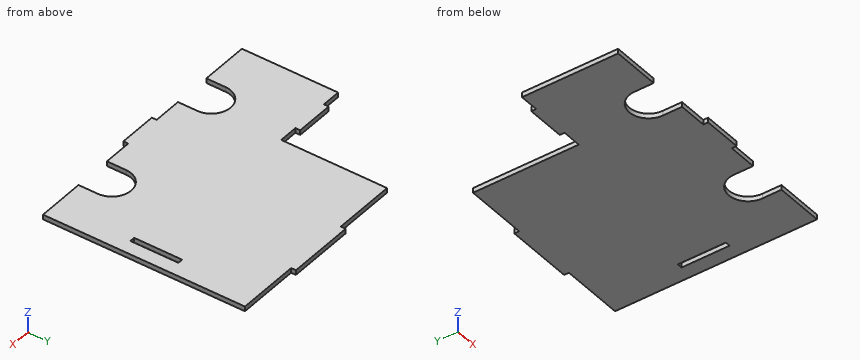
Autodesk Inventor part; units mm, degrees
ref_plane "YZ Plane" through (0, 0, 0) normal (1, 0, 0) x (0, 1, 0)
ref_plane "XZ Plane" through (0, 0, 0) normal (0, 1, 0) x (-1, 0, 0)
ref_plane "XY Plane" through (0, 0, 0) normal (0, 0, 1) x (1, 0, 0)
sketch "Sketch1" plane through (0, 0, 0) normal (0, 0, 1) x (1, 0, 0)
  line L0 (0, 0) -> (0, 100)
  line L1 (0, 100) -> (80, 100)
  line L2 (80, 100) -> (80, 210)
  line L3 (80, 210) -> (280, 210)
  line L4 (280, 210) -> (280, 0)
  line L5 (0, 0) -> (50, 0)
  line L6 (50, 0) -> (50, 20)
  arc A0 (90, 20) -> (50, 20) centre (70, 20) ccw
  line L7 (90, 20) -> (90, 0)
  line L8 (140, 0) -> (140, 210) construction
  line L9 (90, 0) -> (140, 0)
  line L10 (280, 0) -> (230, 0)
  line L11 (230, 0) -> (230, 20)
  arc A1 (230, 20) -> (190, 20) centre (210, 20) ccw
  line L12 (190, 20) -> (190, 0)
  line L13 (190, 0) -> (140, 0)
  line L14 (145, 210) -> (215, 210)
  line L15 (215, 210) -> (215, 215)
  line L16 (215, 215) -> (145, 215)
  line L17 (145, 215) -> (145, 210)
  line L18 (265.3, 80) -> (260, 80)
  line L19 (260, 80) -> (260, 130)
  line L20 (260, 130) -> (265.3, 130)
  line L21 (265.3, 130) -> (265.3, 80)
  line L22 (9.7, 20) -> (15, 20)
  line L23 (15, 20) -> (15, 60)
  line L24 (15, 60) -> (9.7, 60)
  line L25 (9.7, 60) -> (9.7, 20)
  line L26 (20, 100) -> (60, 100)
  line L27 (60, 100) -> (60, 105)
  line L28 (60, 105) -> (20, 105)
  line L29 (20, 105) -> (20, 100)
  line L30 (160, 0) -> (160, -5)
  line L31 (160, -5) -> (120, -5)
  line L32 (120, -5) -> (120, 0)
  dimension "d0" = 100
  dimension "d1" = 80
  dimension "d2" = 110
  dimension "d3" = 200
  dimension "d4" = 50
  dimension "d5" = 20
  dimension "d6" = 40
  dimension "d7" = 70
  dimension "d8" = 5
  dimension "d9" = 5.3
  dimension "d10" = 50
  dimension "d12" = 50
  dimension "d13" = 5.3
  dimension "d14" = 40
  dimension "d17" = 40
  dimension "d18" = 5
  dimension "d19" = 40
  dimension "d20" = 5
  dimension "d21" = 20
extrude "Extrusion1" add sketch "Sketch1" along normal blind 5 contours L0 L1 L2 L3 L4 L10 L11 A1 L12 L13 L9 L7 A0 L6 L5 | L29 L28 L27 L1 | L9 L13 L30 L31 L32 | L17 L16 L15 L3 | L25 L24 L23 L22
properties part number "side"
Design review of the part built by this model. Coordinates are the model's own, in mm. Give positions to 0.01 mm unless a question says otherwise; leave off trailing zeros. Write each loop counter-clockwise with the first axis right and the second up, starting at its lowest first coordinate (ties: lowest second). Pieces come first, ordered by that corner, then holes. Notation, with made-up numbers: (-34, -22) - (3, -22) arc R26 ccw to (3, 4) - close; hole circle Ø7 at (14.25, -24.75). An arc over 180 degrees is marked (long way). Return JSON: item names as keys, results as strings. Group by question number.
(1) We need section C-C, the plane x = 35. Give the boundary of the cut face in (y, z), then the cut area to 3 significant figures.
(2) We need section D-D, the plane y = 173. Give the boundary of the cut face in (x, z).
(3) To check wall thickness, follow probe 1 along X at (y, z) = (93, 4.2); probe 2 along X at (y, z) = (28, 1.7); probe 3 along Y at (x, z) = (240, 1.5). State the ranges of each line that lie inside material, in increasing order.
(4) Insertion check: pin 1 (1.5 mm diameter, centred on x = 17, z = 2.5, fed in from -Y); pin 2 (2.5 mm diameter, centred on y = 213, z = 2.5, fed in from -X); pin 3 (1.5 mm diameter, centred on y = -1.5, z = 3, fed in from -X). Each pin has a flat end and moves straight along its axis. Give the tip position at first contact, or say it passes through.
(5) We need section A-A, the plane y = 116.5. Give the boundary of the cut face in (x, z).
Reported:
{
 "1": {"outline": "(0, 0) - (105, 0) - (105, 5) - (0, 5) - close", "area": "525 mm2"},
 "2": {"outline": "(80, 0) - (280, 0) - (280, 5) - (80, 5) - close"},
 "3": {"probe 1": "x = 0 to 260, 265.3 to 280", "probe 2": "x = 0 to 51.67, 88.33 to 191.67, 228.33 to 280", "probe 3": "y = 0 to 210"},
 "4": {"pin 1": "stops at y = 0", "pin 2": "stops at x = 145", "pin 3": "stops at x = 120"},
 "5": {"outline": "(80, 0) - (260, 0) - (260, 5) - (80, 5) - close; (265.3, 0) - (280, 0) - (280, 5) - (265.3, 5) - close"}
}
